Design review of the part built by this model. Coordinates are the model's own, in mm. A direction names the side the tool comes from. Round coordinates to 2 decimals unless told otherwise and drop trailing zeros. Loops run counter-clockwise (first coordinate to the right, second up) from the corner with the lowest first, then second, coordinate; pieces in that order, holes last. Notation, with made-up numbers: (2, -19) - (14, -19) arc R13 cw to (14, 0) - close; hole circle Ø9 at (14.25, 53). An arc over 180 degrees is marked (long way). Answer as CSV lines item,"result". Start each with the question number.
(1) For faces 4 (the flat face through (-94, 94, -3)), 5 (the flat face through (-2, 139.5, 4)), 6 (the flat face through (14, 151, 7)), 7 (the flat face through (-14, 151, 7)), 8 (the flat face through (-3, 135.5, 9)), list the 3-axis set-ups (+Z, -Z, +X, -X, +Y, -Y) from which the entire face can be reached by the end or side of a thin tool; tool diameter is ignored.
(2) Consider section A-A (x = 0). Give the boundary of the cut face in (y, z), and give its area (3 significant figures).
(3) Wall thickness on L1, parallel to Z at x = -11.3, y = 149.5; L2, parallel to Z at x = -25, y = 149; L3, parallel to X at y = 153, z = 11.5: over which ranges is each line inside the solid? List them lowest first.
(4) For P1, Ø5, axis at x = 38.5, y = 144, coming from the +Z side; P2, Ø10, axis at x = -0.5, z = 9, coming from the +Y side; P3, Ø8, axis at x = -16, z = 13, coming from the -Y side; P4, Ø9, axis at y = 149.5, z = 10, coming from the +X side, all flat-tipped, find the tip position at first contact; note any pin that passes through.
(5) Mouldability with a two-part tool opening along X and no side actions: class faces 1 (the flat face through (0, 130, -6.1)), 2 (the flat face through (-70.232, 109.373, -3.007)), 3 (the cylindrical face through (-87.41, 109.36, -3.01)) as released by +X, released by -X, zero draft, split by the parting line, or undercut.
(6) Consider section D-D (y = 131.5). Give the boundary of the cut face in (x, z), and give its area (3 significant figures).
(7) Consider section B-B (y = 149.5). Give the boundary of the cut face in (x, z), and give its area (3 significant figures).
(8) Consider section C-C (y = 104.5). Give the boundary of the cut face in (x, z), and give its area (3 significant figures).
from build123d import *

# Parameters (mm, degrees)
BOSS_EXTRUDE4_DEPTH     = 6.1
BOSS_EXTRUDE5_DEPTH     = 20
BOSS_EXTRUDE6_DEPTH     = 6.1
BOSS_EXTRUDE7_DEPTH     = 20
CUT_EXTRUDE1_DEPTH      = 189.786254796
CUT_EXTRUDE1_DEPTH_BACK = 189.786254796
SKETCH9_W               = 20.1
SKETCH9_H               = 10
SKETCH10_R              = 2.75
CUT_EXTRUDE2_DEPTH      = 20
SKETCH11_R              = 6
CUT_EXTRUDE3_DEPTH      = 4
CUT_EXTRUDE4_DEPTH      = 189.786254796
CUT_EXTRUDE4_DEPTH_BACK = 189.786254796
SKETCH12_R              = 2.75
SKETCH13_R              = 6
CUT_EXTRUDE5_DEPTH      = 197.489461759
SKETCH14_R              = 6
CUT_EXTRUDE6_DEPTH      = 197.489461759


with BuildPart() as part:
    # Sketch5 → Boss-Extrude4 (new body)
    with BuildSketch(Plane.XY):
        with BuildLine():
            Line((-89.802561211, 89.802561211), (-50.105122421, 129.5))
            Line((-50.105122421, 129.5), (50.105122421, 129.5))
            Line((50.105122421, 129.5), (89.802561211, 89.802561211))
            Line((89.802561211, 89.802561211), (98.994949366, 98.994949366))
            ThreePointArc((98.994949366, 98.994949366), (0, 140), (-98.994949366, 98.994949366))
            Line((-98.994949366, 98.994949366), (-89.802561211, 89.802561211))
        make_face()
    extrude(amount=-BOSS_EXTRUDE4_DEPTH)

    # Sketch6 → Boss-Extrude5 (add)
    with BuildSketch(Plane.XY):
        Polygon((10.05, 139.5), (-10.05, 139.5), (-10.05, 159.5), (-50.105122421, 130.726725298), (-50.105122421, 129.5), (50.105122421, 129.5), (50.105122421, 130.726725298), (10.05, 159.5), align=None)
    extrude(amount=BOSS_EXTRUDE5_DEPTH)

    # Sketch7 → Boss-Extrude6 (add)
    with BuildSketch(Plane.XY):
        with BuildLine():
            Line((-10.05, 159.5), (-75.100690367, 118.15196277))
            ThreePointArc((-75.100690367, 118.15196277), (-87.573230694, 109.228793209), (-98.994949366, 98.994949366))
            Line((-98.994949366, 98.994949366), (-89.802561211, 89.802561211))
            Line((-89.802561211, 89.802561211), (-50.105122421, 129.5))
            Line((-50.105122421, 129.5), (50.105122421, 129.5))
            Line((50.105122421, 129.5), (89.802561211, 89.802561211))
            Line((89.802561211, 89.802561211), (98.994949366, 98.994949366))
            ThreePointArc((98.994949366, 98.994949366), (87.573230694, 109.228793209), (75.100690367, 118.15196277))
            Line((75.100690367, 118.15196277), (10.05, 159.5))
            Line((10.05, 159.5), (10.05, 139.5))
            Line((10.05, 139.5), (-10.05, 139.5))
            Line((-10.05, 139.5), (-10.05, 159.5))
        make_face()
    extrude(amount=-BOSS_EXTRUDE6_DEPTH)

    # Sketch8 → Boss-Extrude7 (add)
    with BuildSketch(Plane.XY):
        Polygon((-50.105122421, 130.726725298), (-50.105122421, 129.5), (-57.247420766, 129.5), (-10.05, 159.5), align=None)
        Polygon((50.105122421, 129.5), (57.247420766, 129.5), (10.05, 159.5), (50.105122421, 130.726725298), align=None)
    extrude(amount=BOSS_EXTRUDE7_DEPTH)

    # Sketch9 → Cut-Extrude1 (cut, two sides: drawn at the far end of the back side and taken through both)
    with BuildSketch(Plane.XY.offset(-CUT_EXTRUDE1_DEPTH_BACK)):
        with Locations((0, 144.5)):
            Rectangle(SKETCH9_W, SKETCH9_H)
    extrude(amount=CUT_EXTRUDE1_DEPTH + CUT_EXTRUDE1_DEPTH_BACK, mode=Mode.SUBTRACT)

    # Sketch10 → Cut-Extrude2 (cut)
    with BuildSketch(Plane(origin=(0, 139.5, 0), x_dir=(1, 0, 0), z_dir=(0, 1, 0))):
        with Locations(Location((0, -10, 0), (0, 0, 180))):
            Circle(SKETCH10_R)
    extrude(amount=-CUT_EXTRUDE2_DEPTH, mode=Mode.SUBTRACT)

    # Sketch11 → Cut-Extrude3 (cut)
    with BuildSketch(Plane(origin=(0, 139.5, 0), x_dir=(1, 0, 0), z_dir=(0, 1, 0))):
        with Locations(Location((0, -10, 0), (0, 0, 180))):
            Circle(SKETCH11_R)
    extrude(amount=-CUT_EXTRUDE3_DEPTH, mode=Mode.SUBTRACT)

    # Sketch12 → Cut-Extrude4 (cut, two sides: drawn at the far end of the back side and taken through both)
    with BuildSketch(Plane(origin=(0, 0, 0), x_dir=(0, 0, -1), z_dir=(1, 0, 0)).offset(-CUT_EXTRUDE4_DEPTH_BACK)):
        with Locations(Location((-10, 149.5, 0), (0, 0, 270))):
            Circle(SKETCH12_R)
    extrude(amount=CUT_EXTRUDE4_DEPTH + CUT_EXTRUDE4_DEPTH_BACK, mode=Mode.SUBTRACT)

    # Sketch13 → Cut-Extrude5 (cut, through all)
    with BuildSketch(Plane(origin=(14, 0, 0), x_dir=(0, 0, -1), z_dir=(1, 0, 0))):
        with Locations(Location((-10, 149.5, 0), (0, 0, 90))):
            Circle(SKETCH13_R)
    extrude(amount=CUT_EXTRUDE5_DEPTH, mode=Mode.SUBTRACT)

    # Sketch14 → Cut-Extrude6 (cut, through all)
    with BuildSketch(Plane(origin=(-14, 0, 0), x_dir=(0, 0, -1), z_dir=(1, 0, 0))):
        with Locations(Location((-10, 149.5, 0), (0, 0, 90))):
            Circle(SKETCH14_R)
    extrude(amount=-CUT_EXTRUDE6_DEPTH, mode=Mode.SUBTRACT)


solid = part.part
Determined:
1,face 4,"+Z, -Z, -X, -Y"
1,face 5,"+Z, -Z, +Y"
1,face 6,"+X"
1,face 7,"-X"
1,face 8,"+Y"
2,outline,"(129.5, -6.1) - (139.5, -6.1) - (139.5, 4) - (135.5, 4) - (135.5, 7.25) - (129.5, 7.25) - close; (129.5, 12.75) - (135.5, 12.75) - (135.5, 16) - (139.5, 16) - (139.5, 20) - (129.5, 20) - close"
2,area,"180 mm^2"
3,L1,"z = -6.1 to 7.25, 12.75 to 20"
3,L2,"z = -6.1 to 4.02, 15.98 to 20"
3,L3,"x = -14 to -10.05, 10.05 to 14"
4,P1,"stops at z = 20"
4,P2,"stops at y = 139.5"
4,P3,"stops at y = 129.5"
4,P4,"stops at x = 14"
5,face 1,"zero draft"
5,face 2,"undercut"
5,face 3,"released by -X"
6,outline,"(-54.1, -6.1) - (54.1, -6.1) - (54.1, 20) - (-54.1, 20) - close; hole circle Ø5.5 at (0, 10)"
6,area,"2,800 mm^2"
7,outline,"(-25.78, -6.1) - (-10.05, -6.1) - (-10.05, 7.25) - (-14, 7.25) - (-14, 4) - (-25.78, 4) - close; (-25.78, 16) - (-14, 16) - (-14, 12.75) - (-10.05, 12.75) - (-10.05, 20) - (-25.78, 20) - close; (10.05, -6.1) - (25.78, -6.1) - (25.78, 4) - (14, 4) - (14, 7.25) - (10.05, 7.25) - close; (10.05, 12.75) - (14, 12.75) - (14, 16) - (25.78, 16) - (25.78, 20) - (10.05, 20) - close"
7,area,"495 mm^2"
8,outline,"(-93.17, -6.1) - (-75.11, -6.1) - (-75.11, 0) - (-93.17, 0) - close; (75.11, -6.1) - (93.17, -6.1) - (93.17, 0) - (75.11, 0) - close"
8,area,"220 mm^2"
